Geometry: final body of the model. Coordinates: model frame, mm. A direction names the side the tool comes from. Give positions to 0.01 mm unless a question says otherwise; leave off trailing zeros. Write each loop counter-clockwise with the first axis right and the second up, starting at its lowest first coordinate (ties: lowest second). Pieces come first, ordered by that corner, then holes.
Q1. Section C-C (z = 20). Return the cut outline in (x, y).
Q2. Mould query, pull axis Z, two halves, no side actions, for faces 1 (the flat face through (0, 3, 18)), 2 (the cylindrical face through (-5.569, 3.131, 20.125)), 3 (the flat face through (-28, 3, 0)). Classes: +Z half, -Z half, draft (parallel to the pull), parting line (faces both ways), or undercut.
Q3. Line query: line 1 (X direction, y = 3.75, z = 16) (3 decimals); line 2 (Z direction, x = -28, y = 2.5) (3 decimals); line 3 (Z direction, x = -15, y = 1.5) (3 decimals). Output: solid intervals per line, ascending.
Q4. Section D-D (y = 1.75). State how many separate pieces and enclosed holes the cut face has, plus the area to 3 significant figures.
Q5. Pin query (flat end, axial travel): pin 1 Ø11 at (x, z) = (-11.11, 15.88) entering from +Y. Return the tip coordinate at first contact, or that it passes through.
Q6. Section B-B (x = -9). Return the cut outline in (y, z) (3 decimals).
Q7. Reachability of faces 4 (the flat face through (-38, 3, 19.05)), 5 (the flat face through (-28, 0, 22)) from +Z, -Z, +X, -X, +Y, -Y: full face, straight path, thin tool, end or side. Return the list, or none.
Q8. Section A-A (z = 15). Return the cut outline in (x, y) (3 decimals), plus the area to 3 significant figures.
Autodesk Inventor part; units mm, degrees
ref_plane "YZ Plane" through (0, 0, 0) normal (1, 0, 0) x (0, 1, 0)
ref_plane "XZ Plane" through (0, 0, 0) normal (0, 1, 0) x (-1, 0, 0)
ref_plane "XY Plane" through (0, 0, 0) normal (0, 0, 1) x (1, 0, 0)
sketch "Sketch1" plane through (0, 0, 0) normal (0, 1, 0) x (-1, 0, 0)
  line L0 (57.15, 34.925) -> (57.15, 0)
  line L1 (57.15, 34.925) -> (0, 34.925)
  line L2 (57.15, 0) -> (57.15, 15.875)
  line L3 (34.925, 12.7) -> (41.275, 12.7)
  line L4 (41.275, 12.7) -> (41.275, 19.05)
  line L5 (41.275, 19.05) -> (34.925, 19.05)
  line L6 (34.925, 19.05) -> (34.925, 12.7)
  line L7 (34.925, 12.7) -> (41.275, 19.05) construction
  line L8 (41.275, 12.7) -> (34.925, 19.05) construction
  line L9 (28.575, 12.7) -> (22.225, 12.7)
  line L10 (22.225, 12.7) -> (22.225, 19.05)
  line L11 (22.225, 19.05) -> (28.575, 19.05)
  line L12 (28.575, 19.05) -> (28.575, 12.7)
  line L13 (28.575, 12.7) -> (22.225, 19.05) construction
  line L14 (22.225, 12.7) -> (28.575, 19.05) construction
  circle A0 centre (11.1125, 15.875) radius 6.985
  line L15 (57.15, 34.925) -> (3.175, 34.925)
  line L16 (3.175, 0) -> (57.15, 0)
  line L17 (57.15, 0) -> (57.15, 34.925)
  line L18 (0, 34.925) -> (0, 0)
  line L19 (0, 0) -> (57.15, 0)
  point P0 (0, 0)
  dimension "d0" = 57.15
  dimension "d1" = 15.875
  dimension "d4" = 6.35
  dimension "d5" = 6.35
  dimension "d6" = 6.35
  dimension "d7" = 6.35
  dimension "d9" = 13.97
  dimension "d11" = 0
  dimension "d12" = 53.975
  dimension "d13" = 57.15
  dimension "d14" = 34.925
  dimension "d15" = 90
  dimension "d16" = 3.175
  dimension "d17" = 12.7
  dimension "d18" = 12.7
  dimension "d19" = 6.35
  dimension "d20" = 15.875
  dimension "d21" = 11.1125
  dimension "d22" = 15.875
  dimension "d23" = 11.1125
  dimension "d24" = 34.925
extrude "Extrusion1" add sketch "Sketch1" along normal blind 6.35
properties part number "RCcar_motor_testplate"
Computed:
1. outline: (-57.15, 0) - (-16.75, 0) - (-16.75, 6.35) - (-57.15, 6.35) - close; (-5.48, 0) - (0, 0) - (0, 6.35) - (-5.48, 6.35) - close
2. face 1: draft
2. face 2: undercut
2. face 3: -Z half
3. line 1: x = -57.15 to -41.275, -34.925 to -28.575, -22.225 to -18.096, -4.129 to 0
3. line 2: z = 0 to 12.7, 19.05 to 34.925
3. line 3: z = 0 to 10.072, 21.678 to 34.925
4. separate pieces: 1
4. enclosed holes: 3
4. area: 1,760 mm2
5. pin 1: passes through
6. outline: (0, 0) - (6.35, 0) - (6.35, 9.217) - (0, 9.217) - close; (0, 22.533) - (6.35, 22.533) - (6.35, 34.925) - (0, 34.925) - close
7. face 4: +Y, -Y
7. face 5: +Z, -Z, +X, -X, -Y
8. outline: (-57.15, 0) - (-41.275, 0) - (-41.275, 6.35) - (-57.15, 6.35) - close; (-34.925, 0) - (-28.575, 0) - (-28.575, 6.35) - (-34.925, 6.35) - close; (-22.225, 0) - (-18.042, 0) - (-18.042, 6.35) - (-22.225, 6.35) - close; (-4.183, 0) - (0, 0) - (0, 6.35) - (-4.183, 6.35) - close
8. area: 194 mm2
